CAD build for the part. Positions are in the model's coordinates, mm. A direction names the side the tool comes from. Coordinates: 2 decimals unless noted, no trailing zeros. Loops run counter-clockwise (first coordinate to the right, second up) from the corner with the lowest first, then second, coordinate; pieces in that order, holes last. Notation, with made-up numbers: (75.5, 1) -> (109.5, 1) arc R27 cw to (109.5, 22) -> close; hole circle Ø3 at (44.5, 7.25). An arc over 180 degrees is marked (long way). Return JSON: item names as keys, results as strings. Group by question number.
(1) Saw through at D-D on x = 4. Write the cut outline in (y, z), then the cut area to 3 significant figures.
(2) Saw through at C-C on y = 0.55. Write the cut outline in (x, z), then the cut area to 3 significant figures.
(3) Probe L1, parallel to Z at x = 2.25, y = 1.6; L2, parallel to X at y = 0.3, z = -14; L3, parallel to Y at x = 2.75, z = -1. List the from-to ranges inside material, lowest first.
(4) Saw through at B-B on x = 7.25. Write the cut outline in (y, z).
(5) Mould opens along Z. For faces 3 (the face through (-10.147, 1, -8)), 4 (the face through (5, 1, 6.302)), 5 (the face through (1.745, 1.823, -1.175)) say: pulls with the +Z half, pulls with the -Z half, needs draft (parallel to the pull), parting line crosses it, or undercut.
(6) Tool access for faces 1 (the face through (6.54, 1.82, -2.37)), 2 (the face through (5, 1, 0.302)): list every direction of +Z, -Z, +X, -X, +Y, -Y with a clear straight run to the whole face (end or side of a thin tool).
(7) Saw through at A-A on z = -6.75. Write the cut outline in (x, y), then the cut area to 3 significant figures.
(8) Flat gauge pin, fed straight in: pin 1 Ø10.5 at (x, z) = (4.85, -8.25) entering from -Y. Where does the tip first touch, or does it go through?
```python
from build123d import *

# Parameters (mm, degrees)
BOSS_EXTRUDE1_DEPTH                             = 2
CSK_FOR_M2_FLAT_HEAD_MACHINE_SCREW1_D           = 2.2
CSK_FOR_M2_FLAT_HEAD_MACHINE_SCREW1_DEPTH       = 4
CSK_FOR_M2_FLAT_HEAD_MACHINE_SCREW1_CSINK_D     = 4.4
CSK_FOR_M2_FLAT_HEAD_MACHINE_SCREW1_CSINK_ANGLE = 90
CSK_FOR_M2_FLAT_HEAD_MACHINE_SCREW1_TIP         = 0.660946681
SKETCH9_W                                       = 11.5
SKETCH9_H                                       = 17.1
CUT_EXTRUDE1_DEPTH                              = 1.651
SKETCH11_R                                      = 4.572
SKETCH11_R_2                                    = 1.524
CUT_EXTRUDE2_DEPTH                              = 31.275155769


with BuildPart() as part:
    # Sketch1 → Boss-Extrude1 (new body)
    with BuildSketch(Plane(origin=(0, 0, 0), x_dir=(1, 0, 0), z_dir=(0, 1, 0))):
        Polygon((-10.147286186, 19.79756588), (-10.147286186, -3.30243412), (-6.697286186, -6.30243412), (16.402713814, -6.30243412), (19.852713814, -3.30243412), (19.852713814, 19.79756588), (16.402713814, 22.79756588), (-6.697286186, 22.79756588), align=None)
    extrude(amount=BOSS_EXTRUDE1_DEPTH)

    # CSK for M2 Flat Head Machine Screw1
    with Locations(Plane(origin=(0, 2, 0), x_dir=(1, 0, 0), z_dir=(0, 1, 0))):
        with Locations((-7.347286186, 15.79756588), (17.052713814, 15.79756588), (17.052713814, 0.69756588), (-7.347286186, 0.69756588)):
            CounterSinkHole(CSK_FOR_M2_FLAT_HEAD_MACHINE_SCREW1_D / 2, CSK_FOR_M2_FLAT_HEAD_MACHINE_SCREW1_CSINK_D / 2, depth=CSK_FOR_M2_FLAT_HEAD_MACHINE_SCREW1_DEPTH, counter_sink_angle=CSK_FOR_M2_FLAT_HEAD_MACHINE_SCREW1_CSINK_ANGLE)
            with Locations((0, 0, -(CSK_FOR_M2_FLAT_HEAD_MACHINE_SCREW1_DEPTH + CSK_FOR_M2_FLAT_HEAD_MACHINE_SCREW1_TIP / 2))):  # 118° drill point
                Cone(0, CSK_FOR_M2_FLAT_HEAD_MACHINE_SCREW1_D / 2, CSK_FOR_M2_FLAT_HEAD_MACHINE_SCREW1_TIP, mode=Mode.SUBTRACT)

    # Sketch9 → Cut-Extrude1 (cut)
    with BuildSketch(Plane(origin=(0, 0, 0), x_dir=(1, 0, 0), z_dir=(0, 1, 0))):
        with Locations((4.852713814, 8.24756588)):
            Rectangle(SKETCH9_W, SKETCH9_H)
    extrude(amount=CUT_EXTRUDE1_DEPTH, mode=Mode.SUBTRACT)

    # Sketch11 → Cut-Extrude2 (cut, through all)
    with BuildSketch(Plane.XZ.offset(-1.651)):
        with Locations(Location((4.852713814, -8.24756588, 0), (0, 0, 270))):
            Circle(SKETCH11_R)
        with Locations(Location((8.027713814, -2.69756588, 0), (0, 0, 270))):
            Circle(SKETCH11_R_2)
        with Locations(Location((1.677713814, -2.69756588, 0), (0, 0, 270))):
            Circle(SKETCH11_R_2)
    extrude(amount=-CUT_EXTRUDE2_DEPTH, mode=Mode.SUBTRACT)


solid = part.part
```
Geometry results:
{
 "1": {"outline": "(0, -22.8) -> (2, -22.8) -> (2, -12.74) -> (1.65, -12.74) -> (1.65, -16.8) -> (0, -16.8) -> close; (0, 0.3) -> (1.65, 0.3) -> (1.65, -3.76) -> (2, -3.76) -> (2, 6.3) -> (0, 6.3) -> close", "area": "26.8 mm²"},
 "2": {"outline": "(-10.15, -19.8) -> (-6.7, -22.8) -> (16.4, -22.8) -> (19.85, -19.8) -> (19.85, 3.3) -> (16.4, 6.3) -> (-6.7, 6.3) -> (-10.15, 3.3) -> close; hole circle Ø2.2 at (-7.35, -15.8); hole circle Ø2.2 at (-7.35, -0.7); hole (-0.9, -16.8) -> (10.6, -16.8) -> (10.6, 0.3) -> (-0.9, 0.3) -> close; hole circle Ø2.2 at (17.05, -15.8); hole circle Ø2.2 at (17.05, -0.7)", "area": "640 mm²"},
 "3": {"L1": "-22.8 to -16.8, 0.3 to 6.3", "L2": "-10.15 to -0.9, 10.6 to 19.85", "L3": "1.65 to 2"},
 "4": {"outline": "(0, -22.8) -> (2, -22.8) -> (2, -12.14) -> (1.65, -12.14) -> (1.65, -16.8) -> (0, -16.8) -> close; (0, 0.3) -> (1.65, 0.3) -> (1.65, -1.39) -> (2, -1.39) -> (2, 6.3) -> (0, 6.3) -> close; (1.65, -4.35) -> (2, -4.35) -> (2, -4.01) -> (1.65, -4.01) -> close"},
 "5": {"face 3": "needs draft", "face 4": "pulls with the +Z half", "face 5": "undercut"},
 "6": {"face 1": "+Y, -Y", "face 2": "-Y"},
 "7": {"outline": "(-10.15, 0) -> (-0.9, 0) -> (-0.9, 1.65) -> (0.53, 1.65) -> (0.53, 2) -> (-10.15, 2) -> close; (9.17, 1.65) -> (10.6, 1.65) -> (10.6, 0) -> (19.85, 0) -> (19.85, 2) -> (9.17, 2) -> close", "area": "38.0 mm²"},
 "8": {"pin 1": "y = 1.65"}
}
